Build history of the part. All positions in model axes, mm. A direction names the side the tool comes from. Round coordinates to 2 decimals unless told otherwise and drop trailing zeros. Write each loop counter-clockwise with the first axis right and the second up, starting at its lowest first coordinate (ties: lowest second). Pieces come first, ordered by that corner, then holes.
Item 1: Band-saw the part on C-C, the plane z = -3.25. Write the cut outline in (x, y).
Item 2: Band-saw the part on A-A, the plane y = 5. Write the cut outline in (x, z).
Item 3: Mould opens along Y. For faces 1 (the flat face through (-4.5, 0, -0.1)), 2 (the cylindrical face through (-1.11, 16.01, 4.51)), 3 (the flat face through (-4.5, 58, -0.1)) say: +Y half, -Y half, draft (parallel to the pull), parting line (faces both ways), or undercut.
Item 4: Band-saw the part on D-D, the plane x = 3. Write the cut outline in (y, z), then the cut area to 3 significant figures.
Item 5: Band-saw the part on B-B, the plane y = 24. Write the cut outline in (x, z).
Item 6: Drop a flat-ended pin along its axis: pin 1 Ø4 at (x, y) = (0, 15) entering from -Z. Give the stop position or say it passes through.
Item 7: Wall check: probe 1 along Y at (x, z) = (0, 4.6); probe 2 along Z at (x, y) = (1.5, 49). Give the ranges that are in metal, low to high.
Item 8: 3-axis set-ups, long thin cutter, end or side, ignore diameter. For faces 4 (the flat face through (0, 29, 4)), 5 (the cylindrical face through (-4.507, 30.487, -0.195)): which of +Z, -Z, +X, -X, +Y, -Y reach the whole face in a straight line?
```python
from build123d import *

# Parameters (mm, degrees)
SKETCH_1_W          = 10
SKETCH_1_H          = 10
SKETCH_1_W_2        = 8
SKETCH_1_H_2        = 8
EXTRUDE_1_DEPTH     = 58
SKETCH_2_R          = 1.5
CUT_EXTRUDE_1_DEPTH = 30
SKETCH_3_R          = 1.5
CUT_EXTRUDE_2_DEPTH = 30


with BuildPart() as part:
    # 草图1 → 凸台-拉伸1 (new body)
    with BuildSketch(Plane(origin=(0, 0, 0), x_dir=(1, 0, 0), z_dir=(0, 1, 0))):
        Rectangle(SKETCH_1_W, SKETCH_1_H)
        Rectangle(SKETCH_1_W_2, SKETCH_1_H_2, mode=Mode.SUBTRACT)
    extrude(amount=EXTRUDE_1_DEPTH)

    # 草图2 → 切除-拉伸1 (cut)
    with BuildSketch(Plane.XY.offset(5)):
        with Locations((0, 5)):
            Circle(SKETCH_2_R)
        with Locations((0, 15)):
            Circle(SKETCH_2_R)
    extrude(amount=-CUT_EXTRUDE_1_DEPTH, mode=Mode.SUBTRACT)

    # 草图3 → 切除-拉伸2 (cut)
    with BuildSketch(Plane.ZY.offset(5)):
        with Locations((0, 49)):
            Circle(SKETCH_3_R)
        with Locations((0, 29)):
            Circle(SKETCH_3_R)
    extrude(amount=-CUT_EXTRUDE_2_DEPTH, mode=Mode.SUBTRACT)


solid = part.part
```
Results:
1. outline: (-5, 0) - (-4, 0) - (-4, 58) - (-5, 58) - close; (4, 0) - (5, 0) - (5, 58) - (4, 58) - close
2. outline: (-5, -5) - (-1.5, -5) - (-1.5, -4) - (-4, -4) - (-4, 4) - (-1.5, 4) - (-1.5, 5) - (-5, 5) - close; (1.5, -5) - (5, -5) - (5, 5) - (1.5, 5) - (1.5, 4) - (4, 4) - (4, -4) - (1.5, -4) - close
3. face 1: -Y half
3. face 2: undercut
3. face 3: +Y half
4. outline: (0, -5) - (58, -5) - (58, -4) - (0, -4) - close; (0, 4) - (58, 4) - (58, 5) - (0, 5) - close
4. area: 116 mm2
5. outline: (-5, -5) - (5, -5) - (5, 5) - (-5, 5) - close; hole (-4, -4) - (4, -4) - (4, 4) - (-4, 4) - close
6. pin 1: stops at z = -5
7. probe 1: y = 0 to 3.5, 6.5 to 13.5, 16.5 to 58
7. probe 2: z = -5 to -4, 4 to 5
8. face 4: +Y, -Y
8. face 5: +X, -X
